Part print with two shaded views. Sizes in mm from the minimum x, y, z corner. Give positions to 0.01 mm unless a question says otherwise; leave off trailing zeros. Order: outer loops, then holes, each group sorted by start corner. A loop starts at its lowest first (then second) coordinate and runs counter-clockwise, first axis right, second up.
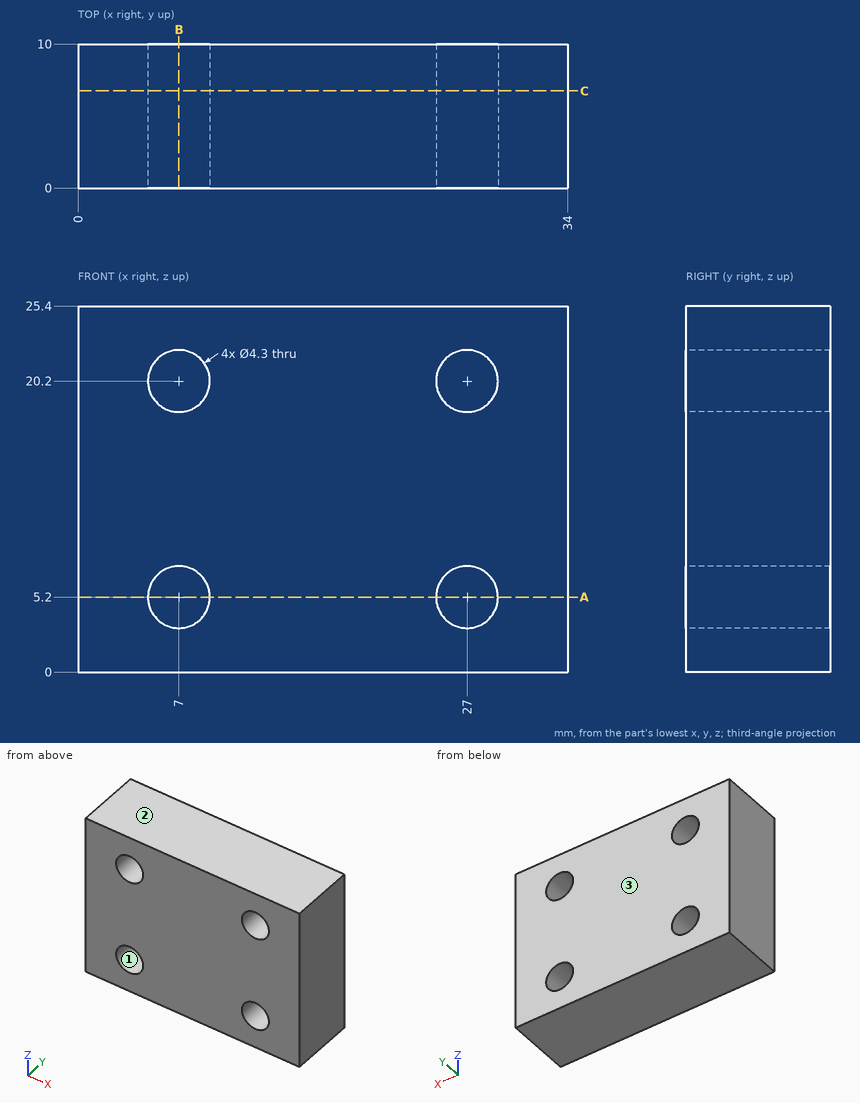
1. Saw through at C-C on y = 6.75. Give the cut face in (x, z), plus the area to 3 significant figures.
2. Saw through at A-A on z = 5.2. Give the cut face in (x, y), plus the area to 3 significant figures.
3. Wall check: line 1 (X direction, y = 8.75, z = 20.25); line 2 (Z direction, x = 8, y = 6.5); line 3 (X direction, y = 1, z = 21). Give the ranges that are in metal, low to high.
4. Mould opens along Z. For the marked faces 1, 2 and 3 say: released by +Z, released by -Z, zero draft, split by the parting line, or undercut.
5. Saw through at B-B on x = 7. Give the cut face in (y, z).
Reported:
1. outline: (0, 0) - (34, 0) - (34, 25.4) - (0, 25.4) - close; hole circle Ø4.3 at (7, 5.2); hole circle Ø4.3 at (7, 20.2); hole circle Ø4.3 at (27, 5.2); hole circle Ø4.3 at (27, 20.2)
1. area: 806 mm2
2. outline: (0, 0) - (4.85, 0) - (4.85, 10) - (0, 10) - close; (9.15, 0) - (24.85, 0) - (24.85, 10) - (9.15, 10) - close; (29.15, 0) - (34, 0) - (34, 10) - (29.15, 10) - close
2. area: 254 mm2
3. line 1: x = 0 to 4.85, 9.15 to 24.85, 29.15 to 34
3. line 2: z = 0 to 3.3, 7.1 to 18.3, 22.1 to 25.4
3. line 3: x = 0 to 5, 9 to 25, 29 to 34
4. face 1: undercut
4. face 2: released by +Z
4. face 3: zero draft
5. outline: (0, 0) - (10, 0) - (10, 3.05) - (0, 3.05) - close; (0, 7.35) - (10, 7.35) - (10, 18.05) - (0, 18.05) - close; (0, 22.35) - (10, 22.35) - (10, 25.4) - (0, 25.4) - close
